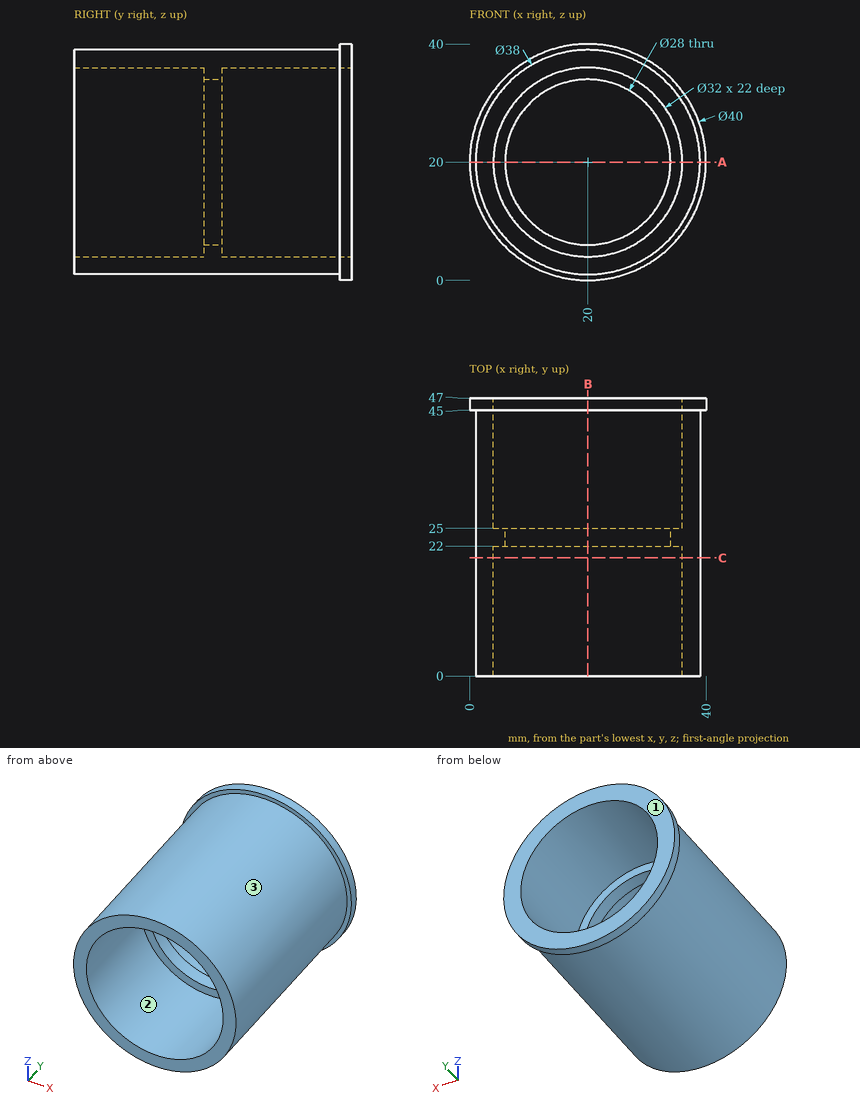
The figure shows three views and two pictorial views of one solid part (mm, origin at its lowest corner). Answer the questions. Give positions to 0.01 mm unless a question says otherwise; leave off trailing zeros. Order: outer loops, then holes, each group sorted by start corner. A loop starts at its lowest first (then second) coordinate and runs counter-clockwise, first axis right, second up. Notation, with made-up numbers: (3.5, -4) -> (28.5, -4) arc R16 ccw to (28.5, 10) -> close; hole circle Ø7 at (17.25, 5). An arc over 180 degrees is marked (long way). Answer as a JSON object with one key per item and string values. Group by question number.
Item 1: Flat-ended cylindrical pins translate along their axes: pin 1 (16 mm diameter, centred on x = 14, z = 16, fed in from -Y); pin 2 (2 mm diameter, centred on x = 26.5, y = 37.5, fed in from +Z); pin 3 (6 mm diameter, centred on x = 21.5, y = 15.5, fed in from +Z). Find the tip coordinate at first contact, or state that the pin passes through.
Item 2: Determine the mould class of the marked faces 1, 2 and 3 for opening direction Z: pulls with the +Z half, pulls with the -Z half, needs draft (parallel to the pull), parting line crosses it, or undercut.
Item 3: The part is cut by section A-A on z = 20. Write down the section's boundary in (x, y).
Item 4: Consider L1, parallel to X at y = 30, z = 20; L2, parallel to X at y = 14, z = 16; L3, parallel to Z at x = 29, y = 41. Determine where each line is inside the solid, lowest interval first. Write a range as from..to.
Item 5: The part is cut by section B-B on x = 20. Write down the section's boundary in (y, z), and give its area (3 significant figures).
Item 6: The part is cut by section C-C on y = 20. Write down the section's boundary in (x, z), and give its area (3 significant figures).
Result set:
{
 "1": {"pin 1": "y = 22", "pin 2": "z = 38.19", "pin 3": "z = 39"},
 "2": {"face 1": "needs draft", "face 2": "undercut", "face 3": "parting line crosses it"},
 "3": {"outline": "(0, 45) -> (1, 45) -> (1, 0) -> (4, 0) -> (4, 22) -> (6, 22) -> (6, 25) -> (4, 25) -> (4, 47) -> (0, 47) -> close; (34, 22) -> (36, 22) -> (36, 0) -> (39, 0) -> (39, 45) -> (40, 45) -> (40, 47) -> (36, 47) -> (36, 25) -> (34, 25) -> close"},
 "4": {"L1": "1..4, 36..39", "L2": "1.43..4.51, 35.49..38.57", "L3": "3.27..6.77, 33.23..36.73"},
 "5": {"outline": "(0, 1) -> (45, 1) -> (45, 0) -> (47, 0) -> (47, 4) -> (25, 4) -> (25, 6) -> (22, 6) -> (22, 4) -> (0, 4) -> close; (0, 36) -> (22, 36) -> (22, 34) -> (25, 34) -> (25, 36) -> (47, 36) -> (47, 40) -> (45, 40) -> (45, 39) -> (0, 39) -> close", "area": "298 mm²"},
 "6": {"outline": "circle Ø38 at (20, 20); hole circle Ø32 at (20, 20)", "area": "330 mm²"}
}
